from build123d import *

# Parameters (mm, degrees)
SKETCH1_W           = 250.19
SKETCH1_H           = 93.472
BOSS_EXTRUDE1_DEPTH = 95.25
SKETCH5_W           = 218.44
SKETCH5_H           = 93.472
CUT_EXTRUDE1_DEPTH  = 79.375
SKETCH6_W           = 15.875
SKETCH6_H           = 25.4
BOSS_EXTRUDE2_DEPTH = 3.175
SKETCH7_R           = 3.937
CUT_EXTRUDE2_DEPTH  = 172.26052419


with BuildPart() as part:
    # Sketch1 → Boss-Extrude1 (new body)
    with BuildSketch(Plane.XY):
        Rectangle(SKETCH1_W, SKETCH1_H)
    extrude(amount=BOSS_EXTRUDE1_DEPTH)

    # Sketch5 → Cut-Extrude1 (cut)
    with BuildSketch(Plane.XY.offset(95.25)):
        Rectangle(SKETCH5_W, SKETCH5_H)
    extrude(amount=-CUT_EXTRUDE1_DEPTH, mode=Mode.SUBTRACT)

    # Sketch6 → Boss-Extrude2 (add)
    with BuildSketch(Plane.XY.offset(95.25)):
        with Locations((117.1575, 59.436)):
            Rectangle(SKETCH6_W, SKETCH6_H)
        with Locations((-117.1575, 59.436)):
            Rectangle(SKETCH6_W, SKETCH6_H)
        with Locations((117.1575, -59.436)):
            Rectangle(SKETCH6_W, SKETCH6_H)
        with Locations((-117.1575, -59.436)):
            Rectangle(SKETCH6_W, SKETCH6_H)
    extrude(amount=-BOSS_EXTRUDE2_DEPTH)

    # Sketch7 → Cut-Extrude2 (cut, through all)
    with BuildSketch(Plane(origin=(0, 0, 92.075), x_dir=(-1, 0, 0), z_dir=(0, 0, -1))):
        with Locations((117.1575, 59.436)):
            Circle(SKETCH7_R)
        with Locations(Location((-117.1575, 59.436, 0), (0, 0, 180))):
            Circle(SKETCH7_R)
        with Locations(Location((117.1575, -59.436, 0), (0, 0, 180))):
            Circle(SKETCH7_R)
        with Locations((-117.1575, -59.436)):
            Circle(SKETCH7_R)
    extrude(amount=-CUT_EXTRUDE2_DEPTH, mode=Mode.SUBTRACT)


solid = part.part
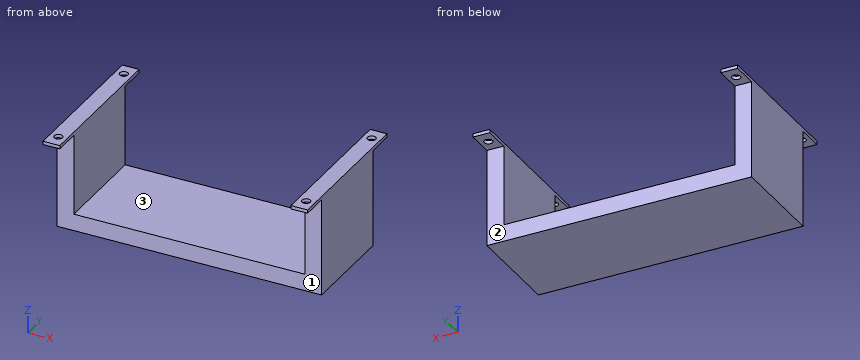
Work out the finished part from the listing and answer in its coordinate system (mm). Face numbers are marked on the shaded views. A direction names the side the tool comes from. Coordinates: 2 decimals unless noted, no trailing zeros. Loops run counter-clockwise (first coordinate to the right, second up) from the corner with the lowest first, then second, coordinate; pieces in that order, holes last. Notation, with made-up numbers: M -7.5,-9 L 31.5,-9 A30 ccw 31.5,24 Z; hole C 54.25,-6.5 d7. An arc over 180 degrees is marked long. Answer in a Markdown table with one row per item. Add a question column.
1. A tool of negligible diameter and unlimited length cuts with its end or side. For the marked faces 1, 2 and 3, from which of +Z, -Z, +X, -X, +Y, -Y can it reach the whole face along a straight path? Write none if from no direction.
2. Find section A-A, the plane z = 47. Write down the section's boundary in (x, y) (3 decimals).
3. Find section B-B, the plane y = 0.5. Write down the section's boundary in (x, z) (3 decimals).
4. Consider L1, parallel to X at y = 24, z = 53 (3 decimals); L2, parallel to Z at x = 76, y = 42 (3 decimals); L3, parallel to Y at x = -71, z = 12. Determine where each line is inside the solid, lowest interval first.
5. Find section C-C, the plane x = -73.5. Write down the section's boundary in (y, z) (3 decimals), then the cut area to 3 significant figures.
6. Flat-ended cylindrical pins translate along their axes: P1, Ø9, axis at x = 117.16, y = -59.44, coming from the -Z side (3 decimals); P2, Ø2, axis at x = 65, y = -11.5, coming from the +Z side (3 decimals); P3, Ø7, axis at x = -117.16, y = 59.44, coming from the +Z side. Find the tip coordinate at first contact, or state that the pin passes through.
Reported:
| question | item | result |
|---|---|---|
| 1 | face 1 | -Z, +X, -X, -Y |
| 1 | face 2 | -Z, +X, -X, +Y |
| 1 | face 3 | +Z, +Y, -Y |
| 2 | outline | M -125.095,-46.736 L -109.22,-46.736 L -109.22,46.736 L -125.095,46.736 Z; M 109.22,-46.736 L 125.095,-46.736 L 125.095,46.736 L 109.22,46.736 Z |
| 3 | outline | M -125.095,0 L 125.095,0 L 125.095,95.25 L 109.22,95.25 L 109.22,15.875 L -109.22,15.875 L -109.22,95.25 L -125.095,95.25 Z |
| 4 | L1 | x = -125.095 to -109.22, 109.22 to 125.095 |
| 4 | L2 | z = 0 to 15.875 |
| 4 | L3 | y = -46.74 to 46.74 |
| 5 | outline | M -46.736,0 L 46.736,0 L 46.736,15.875 L -46.736,15.875 Z |
| 5 | area | 1,480 mm^2 |
| 6 | P1 | stops at z = 92.075 |
| 6 | P2 | stops at z = 15.875 |
| 6 | P3 | passes through |
